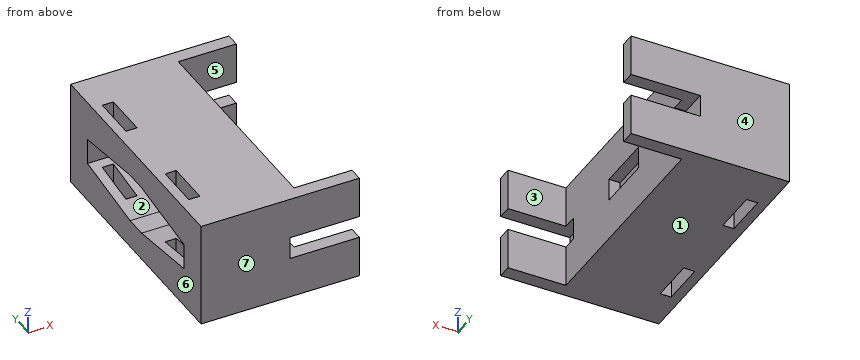
```python
from build123d import *

# Parameters (mm, degrees)
SERVO_CLASPER_2ND_HALF_SERVO_A_DEPTH     = 7.62
VESTIGIAL_START                          = 7.62
CENTER_ENCAPSULATOR_W                    = 2.0574
CENTER_ENCAPSULATOR_H                    = 12.446
CENTER_ENCAPSULATOR_H_2                  = 12.377096657
VESTIGIAL_BUT_NICE_DEPTH                 = 4.1148
SERVO_START                              = 11.7348
SERVO_CLASPER_2ND_HALF_OTHER_SERVO_DEPTH = 7.62
SKETCH12_W                               = 19.3548
SKETCH12_H                               = 45.212
SERVO_HOLDER_EXTRUDE_DEPTH               = 16.350000066
SERVO_B_CUT_DEPTH                        = 7.62
SERVO_B_SECURER_CUT_DEPTH                = 49.176817947
SERVO_B_SECURER_CUT_DEPTH_BACK           = 49.176817947
SKETCH18_W                               = 2.032
SKETCH18_H                               = 8.21582812


with BuildPart() as part:
    # Sketch1 → Servo Clasper 2nd Half (Servo A) (new body)
    with BuildSketch(Plane.XY):
        Polygon((2.60310559, 35.312310559), (2.60310559, 32.772310559), (-8.03949441, 32.772310559), (-8.03949441, -7.359689441), (2.60310559, -7.359689441), (2.60310559, -9.899689441), (-10.09689441, -9.899689441), (-10.09689441, 35.312310559), align=None)
    extrude(amount=SERVO_CLASPER_2ND_HALF_SERVO_A_DEPTH)

    # center encapsulator → Vestigial but nice (add)
    with BuildSketch(Plane.XY.offset(VESTIGIAL_START)):
        with Locations((-9.06819441, 24.072810559)):
            Rectangle(CENTER_ENCAPSULATOR_W, CENTER_ENCAPSULATOR_H)
        with Locations((-9.06819441, 1.374262231)):
            Rectangle(CENTER_ENCAPSULATOR_W, CENTER_ENCAPSULATOR_H_2)
    extrude(amount=VESTIGIAL_BUT_NICE_DEPTH)

    # Sketch7 → Servo Clasper 2nd Half (Other Servo) (add)
    with BuildSketch(Plane.XY.offset(SERVO_START)):
        Polygon((2.60310559, 35.312310559), (2.60310559, 32.772310559), (-8.03949441, 32.772310559), (-8.03949441, -7.359689441), (2.60310559, -7.359689441), (2.60310559, -9.899689441), (-10.09689441, -9.899689441), (-10.09689441, 35.312310559), align=None)
    extrude(amount=SERVO_CLASPER_2ND_HALF_OTHER_SERVO_DEPTH)

    # Sketch12 → Servo Holder Extrude (add)
    with BuildSketch(Plane.ZY.offset(10.09689441)):
        with Locations((9.6774, 12.706310559)):
            Rectangle(SKETCH12_W, SKETCH12_H)
    extrude(amount=SERVO_HOLDER_EXTRUDE_DEPTH)

    # Sketch14 → Servo B Cut (cut)
    with BuildSketch(Plane.ZY.offset(26.446894476)):
        Polygon((7.29615, 29.470310559), (12.05865, 29.470310559), (14.1859, 14.687510559), (14.1859, 10.725110559), (12.05865, -4.057689441), (7.29615, -4.057689441), (5.1689, 10.725110559), (5.1689, 14.687510559), align=None)
    extrude(amount=-SERVO_B_CUT_DEPTH, mode=Mode.SUBTRACT)

    # Sketch18 → Servo B Securer Cut (cut, two sides: drawn at the far end of the back side and taken through both)
    with BuildSketch(Plane(origin=(0, 0, 0), x_dir=(-1, 0, 0), z_dir=(0, 0, -1)).offset(-SERVO_B_SECURER_CUT_DEPTH_BACK)):
        with Locations((23.652894476, 23.584396499)):
            Rectangle(SKETCH18_W, SKETCH18_H)
        Polygon((24.668894476, 5.874578093), (22.636894476, 5.936138467), (22.636894476, -2.279689441), (24.668894476, -2.279689441), align=None)
    extrude(amount=SERVO_B_SECURER_CUT_DEPTH + SERVO_B_SECURER_CUT_DEPTH_BACK, mode=Mode.SUBTRACT)


solid = part.part
```
Build history of the part. All positions in model axes, mm. Face numbers are marked on the shaded views. A direction names the side the tool comes from. Round coordinates to 2 decimals unless told otherwise and drop trailing zeros. Write each loop counter-clockwise with the first axis right and the second up, starting at its lowest first coordinate (ties: lowest second). Pieces come first, ordered by that corner, then holes.
1) Mould opens along Y. For the marked faces 4, 5, 6 and 7 say: +Y half, -Y half, draft (parallel to the pull), parting line (faces both ways), or undercut.
2) Pin check, flat tips, straight feed: pin 1 (1.5 mm diameter, centred on y = 21, z = 5.5, fed in from +X); pin 2 (1 mm diameter, centred on x = -9.5, z = 9.5, fed in from -Y); pin 3 (1 mm diameter, centred on y = 10, z = 8.5, fed in from +X). Stop position of each tip, or through.
3) Band-saw the part on C-C, the plane y = 20.5. List the corners of the cut face in (x, z).
4) 3-axis set-ups, long thin cutter, end or side, ignore diameter. For the marked faces 1, 2 and 3: which of +Z, -Z, +X, -X, +Y, -Y reach the whole face in a straight line?
5) Drill centre lines: probe 1 along Y at (x, z) = (-10, 10.25); probe 2 along Y at (x, z) = (-4, 12.25); probe 3 along X at (y, z) = (4.5, 18.25). Where is each one in solid material? Low to high.
6) Band-saw the part on D-D, the plane z = 10.5. List the corners of the cut face in (x, y).
7) Band-saw the part on B-B, the plane x = -21.75. List the corners of the cut face in (y, z).
8) Band-saw the part on A-A, the plane x = -1.25. List the corners of the cut face in (y, z), and give its area (3 significant figures).
Ans:
1. face 4: +Y half
1. face 5: undercut
1. face 6: draft
1. face 7: -Y half
2. pin 1: stops at x = -8.04
2. pin 2: stops at y = -4.81
2. pin 3: stops at x = -10.1
3. outline: (-26.45, 0) - (-24.67, 0) - (-24.67, 6.01) - (-26.45, 6.01) - close; (-26.45, 13.35) - (-24.67, 13.35) - (-24.67, 19.35) - (-26.45, 19.35) - close; (-22.64, 0) - (-8.04, 0) - (-8.04, 19.35) - (-22.64, 19.35) - (-22.64, 13.35) - (-18.83, 13.35) - (-18.83, 6.01) - (-22.64, 6.01) - close
4. face 1: -Z, +X, -X, +Y, -Y
4. face 2: -X
4. face 3: +Z, -Z, +X
5. probe 1: y = -4.81 to 7.56, 17.85 to 30.3
5. probe 2: y = -9.9 to -7.36, 32.77 to 35.31
5. probe 3: x = -26.45 to -24.67, -22.64 to -8.04
6. outline: (-26.45, -9.9) - (-10.1, -9.9) - (-10.1, -4.81) - (-8.04, -4.81) - (-8.04, 7.56) - (-10.1, 7.56) - (-10.1, 17.85) - (-8.04, 17.85) - (-8.04, 30.3) - (-10.1, 30.3) - (-10.1, 35.31) - (-26.45, 35.31) - (-26.45, 29.47) - (-18.83, 29.47) - (-18.83, -4.06) - (-26.45, -4.06) - close
7. outline: (-9.9, 0) - (35.31, 0) - (35.31, 19.35) - (-9.9, 19.35) - close; hole (-4.06, 7.3) - (10.73, 5.17) - (14.69, 5.17) - (29.47, 7.3) - (29.47, 12.06) - (14.69, 14.19) - (10.73, 14.19) - (-4.06, 12.06) - close
8. outline: (-9.9, 0) - (-7.36, 0) - (-7.36, 7.62) - (-9.9, 7.62) - close; (-9.9, 11.73) - (-7.36, 11.73) - (-7.36, 19.35) - (-9.9, 19.35) - close; (32.77, 0) - (35.31, 0) - (35.31, 7.62) - (32.77, 7.62) - close; (32.77, 11.73) - (35.31, 11.73) - (35.31, 19.35) - (32.77, 19.35) - close
8. area: 77.4 mm2
